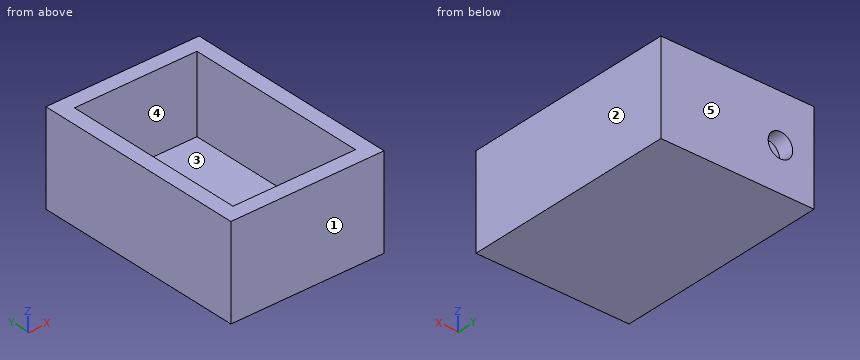
from build123d import *

# Parameters (mm, degrees)
F0_W     = 50
F0_H     = 70
F0_W_2   = 40
F0_H_2   = 60
F1_DEPTH = 30
F2_W     = 40
F2_H     = 60
F3_DEPTH = 25
F4_R     = 4
F5_DEPTH = 5


with BuildPart() as f1:
    # F0 (on Top) → F1 (new body)
    with BuildSketch(Plane.XY):
        Rectangle(F0_W, F0_H)
        Rectangle(F0_W_2, F0_H_2, mode=Mode.SUBTRACT)
        Rectangle(F0_W_2, F0_H_2)
    extrude(amount=F1_DEPTH)

    # F2 (on face) → F3 (cut)
    with BuildSketch(Plane.XY.offset(30)):
        Rectangle(F2_W, F2_H)
    extrude(amount=-F3_DEPTH, mode=Mode.SUBTRACT)

    # F4 (on face) → F5 (cut, through all)
    with BuildSketch(Plane(origin=(0, 35, 0), x_dir=(-1, 0, 0), z_dir=(0, 1, 0))):
        with Locations((14.030943, 14.175501)):
            Circle(F4_R)
    extrude(amount=-F5_DEPTH, mode=Mode.SUBTRACT)


solid = f1.part
The model under review builds one solid part; all positions refer to its coordinate system, in mm. Face numbers are marked on the shaded views. A direction names the side the tool comes from. Give positions to 0.01 mm unless a question says otherwise; leave off trailing zeros. Order: outer loops, then holes, each group sorted by start corner. A loop starts at its lowest first (then second) coordinate and runs counter-clockwise, first axis right, second up. Notation, with made-up numbers: (41, 33) -> (52, 33) arc R14 ccw to (52, 42) -> close; hole circle Ø8 at (-8, 0). An arc over 180 degrees is marked (long way). Write item = value, one per line. Start each with the question number.
(1) Take a section at B-B (x = 15). Write out the cut boundary in (y, z), plus the area to 3 significant figures.
(2) Tool access review of the marked faces 4 and 5: name each direction out of +Z, -Z, +X, -X, +Y, -Y from which nothing blocks a thin tool from reaching the whole face with its end or side.
(3) Draft analysis for pull direction X (two halves, no side actions). For the marked faces 1, 2 and 3, state which applies: +X half, -X half, draft (parallel to the pull), parting line (faces both ways), or undercut.
(4) Take a section at D-D (z = 16). Write out the cut boundary in (x, y), plus the area to 3 significant figures.
(5) Take a section at A-A (z = 23). Write out the cut boundary in (x, y).
(6) For pin 1 Ø5 at (x, z) = (-14.03, 14.18) entering from +Y; pin 2 Ø4 at (x, y) = (-10, 4.5) entering from +Z, all flat-tipped, find the tip position at first contact; note any pin that passes through.
(7) Take a section at C-C (y = 28.5). Write out the cut boundary in (x, z), plus the area to 3 significant figures.
(8) For L1, parallel to X at y = -26.5, z = 27.25; L2, parallel to Y at x = 0.5, z = 10; L3, parallel to Z at x = -7, y = 25, list the stretches that pass through material, from the lowest coordinate up. Write a range as from..to.
Returned:
q1.outline = (-35, 0) -> (35, 0) -> (35, 30) -> (30, 30) -> (30, 5) -> (-30, 5) -> (-30, 30) -> (-35, 30) -> close
q1.area = 600 mm²
q2.face_4 = +Z
q2.face_5 = +Z, -Z, +X, -X, +Y
q3.face_1 = draft
q3.face_2 = +X half
q3.face_3 = undercut
q4.outline = (-25, -35) -> (25, -35) -> (25, 35) -> (-10.47, 35) -> (-10.47, 30) -> (20, 30) -> (20, -30) -> (-20, -30) -> (-20, 30) -> (-17.59, 30) -> (-17.59, 35) -> (-25, 35) -> close
q4.area = 1,060 mm²
q5.outline = (-25, -35) -> (25, -35) -> (25, 35) -> (-25, 35) -> close; hole (-20, -30) -> (20, -30) -> (20, 30) -> (-20, 30) -> close
q6.pin_1 = -30
q6.pin_2 = 5
q7.outline = (-25, 0) -> (25, 0) -> (25, 30) -> (20, 30) -> (20, 5) -> (-20, 5) -> (-20, 30) -> (-25, 30) -> close
q7.area = 500 mm²
q8.L1 = -25..-20, 20..25
q8.L2 = -35..-30, 30..35
q8.L3 = 0..5
